Input: part model. Units: mm. Frame: model coordinates. A direction names the side the tool comes from. Round coordinates to 2 decimals unless told otherwise and drop trailing zeros. Loops run counter-clockwise (first coordinate to the right, second up) from the corner with the lowest first, then second, coordinate; pieces in that order, holes last. Notation, with made-up numbers: (50, 88) -> (86, 88) arc R20 ccw to (86, 99) -> close; hole circle Ø3 at (9, 53). An arc over 180 degrees is marked (long way). Answer as a JSON object with one key per item and string values.
Autodesk Inventor part; units mm, degrees
ref_plane "작업 평면1" through (0, 6, 0) normal (0, 1, 0) x (-1, 0, 0)
ref_plane "YZ Plane" through (0, 0, 0) normal (1, 0, 0) x (0, 1, 0)
ref_plane "XY Plane" through (0, 0, 0) normal (0, 0, 1) x (1, 0, 0)
sketch "스케치1" plane through (0, 0, 0) normal (0, 0, 1) x (1, 0, 0)
  circle A0 centre (0, 0) radius 4
  circle A1 centre (0, 0) radius 6
  circle A2 centre (0, 0) radius 1.9
  dimension "d0" = 8
  dimension "d1" = 2
  dimension "d11" = 3.8
extrude "돌출1" add sketch "스케치1" along normal blind 1 contours A0 | A1
extrude "돌출2" add sketch "스케치1" against normal blind 5 contours A1
ref_plane "작업 평면1" through (0, 6, 0) normal (0, 1, 0) x (-1, 0, 0)
sketch "스케치2" plane through (0, 6, 0) normal (0, 1, 0) x (-1, 0, 0)
  circle A0 centre (0, -2) radius 1
  line L0 (-6, -5) -> (6, -5)
  line L1 (-4, 0) -> (4, 0)
  point P0 (0, 0)
  dimension "d6" = 2
  dimension "d10" = 2
extrude "돌출3" cut sketch "스케치2" against normal through all
chamfer "모따기1" distance 1 angle 45 1 edges at (-6, 0, 1)
fillet "모깎기1" radius 1 1 edges at (-6, 0, -5)
properties part number "SuspensionLock"
1) Draft query along X for faces 1 (the face through (-1.301, -5.857, -1.972)), 2 (the face through (2.2, 0.1, 1)), 3 (the face through (-1.9, -0.08, 0.49)). Return one class per face: +X half, -X half, draft (parallel to the pull), parting line (faces both ways), or undercut.
Output:
{"face 1": "parting line", "face 2": "draft", "face 3": "undercut"}
2) Contact query for flat-ended pins moving along their axis: P1, Ø3, axis at x = -1.5, z = -4.5, coming from the -Y side; P2, Ø2, axis at y = -1.5, z = -1, coming from the -X side; P3, Ø1.2, axis at x = 0, z = -2, coming from the +Y side; P4, Ø1.5, axis at y = 2.5, z = -2.5, coming from the +X side. Output: stop coordinate, or through.
Output:
{"P1": "stops at y = -6", "P2": "stops at x = -5.98", "P3": "passes through", "P4": "stops at x = 5.74"}
3) Section B-B, the plane z = -2.75. Output: boundary loops of the cut face in (x, y).
Output:
{"outline": "(-0.66, -5.96) -> (-0.66, -3.94) arc R4 cw to (-0.66, 3.94) -> (-0.66, 5.96) arc R6 ccw to start; (0.66, -5.96) arc R6 ccw to (0.66, 5.96) -> (0.66, 3.94) arc R4 cw to (0.66, -3.94) -> close"}
4) Section C-C, the plane x = 0. Output: boundary loops of the cut face in (y, z), plus the area to 3 significant figures.
Output:
{"outline": "(-6, -4) arc R1 ccw to (-5, -5) -> (-4, -5) -> (-4, -3) -> (-6, -3) -> close; (-6, -1) -> (-4, -1) -> (-4, 0) -> (-1.9, 0) -> (-1.9, 1) -> (-5, 1) -> (-6, 0) -> close; (1.9, 0) -> (4, 0) -> (4, -1) -> (6, -1) -> (6, 0) -> (5, 1) -> (1.9, 1) -> close; (4, -5) -> (5, -5) arc R1 ccw to (6, -4) -> (6, -3) -> (4, -3) -> close", "area": "18.8 mm^2"}
5) Section D-D, the plane z = -0.75. Output: boundary loops of the cut face in (x, y).
Output:
{"outline": "circle Ø12 at (0, 0); hole circle Ø8 at (0, 0)"}
6) Reachability of faces 4 (the face through (2, -1, 0)), 5 (the face through (-1, -5, -2)) from +Z, -Z, +X, -X, +Y, -Y: full face, straight path, thin tool, end or side. Return the list, or none.
Output:
{"face 4": "-Z", "face 5": "+Y, -Y"}
7) Ray query, probe 1 along Z at (x, y) = (-0.25, 3); probe 2 along Y at (x, z) = (0, 0.7); probe 3 along Z at (x, y) = (0, 4.9). Return the intervals inside material, ascending.
Output:
{"probe 1": "z = 0 to 1", "probe 2": "y = -5.3 to -1.9, 1.9 to 5.3", "probe 3": "z = -5 to -3, -1 to 1"}
8) Section A-A, the plane y = 0. Output: boundary loops of the cut face in (x, z), plus the area to 3 significant figures.
Output:
{"outline": "(-6, -4) arc R1 ccw to (-5, -5) -> (-4, -5) -> (-4, 0) -> (-1.9, 0) -> (-1.9, 1) -> (-5, 1) -> (-6, 0) -> close; (1.9, 0) -> (4, 0) -> (4, -5) -> (5, -5) arc R1 ccw to (6, -4) -> (6, 0) -> (5, 1) -> (1.9, 1) -> close", "area": "26.8 mm^2"}
